from build123d import *

# Parameters (mm, degrees)
F1_DEPTH = 40
F3_DEPTH = 360
F4_R     = 5


with BuildPart() as f1:
    # F0 (on Top) → F1 (new body)
    with BuildSketch(Plane.XY):
        with BuildLine():
            Line((174.920015, 267.026268), (-145.079985, 267.026268))
            ThreePointArc((-145.079985, 267.026268), (-173.364256, 255.310539), (-185.079985, 227.026268))
            Line((-185.079985, 227.026268), (-185.079985, -92.973732))
            ThreePointArc((-185.079985, -92.973732), (-173.364256, -121.258003), (-145.079985, -132.973732))
            Line((-145.079985, -132.973732), (174.920015, -132.973732))
            ThreePointArc((174.920015, -132.973732), (203.204286, -121.258003), (214.920015, -92.973732))
            Line((214.920015, -92.973732), (214.920015, 227.026268))
            ThreePointArc((214.920015, 227.026268), (203.204286, 255.310539), (174.920015, 267.026268))
        make_face()
    extrude(amount=F1_DEPTH)

    # F2 (on face) → F3 (join)
    with BuildSketch(Plane(origin=(0, 0, 0), x_dir=(1, 0, 0), z_dir=(0, 0, -1))):
        with BuildLine():
            ThreePointArc((-145.079985, 62.973732), (-142.151053, 55.902664), (-135.079985, 52.973732))
            Line((-135.079985, 52.973732), (-115.079985, 52.973732))
            ThreePointArc((-115.079985, 52.973732), (-108.008917, 55.902664), (-105.079985, 62.973732))
            Line((-105.079985, 62.973732), (-105.079985, 82.973732))
            ThreePointArc((-105.079985, 82.973732), (-108.008917, 90.0448), (-115.079985, 92.973732))
            Line((-115.079985, 92.973732), (-135.079985, 92.973732))
            ThreePointArc((-135.079985, 92.973732), (-142.151053, 90.0448), (-145.079985, 82.973732))
            Line((-145.079985, 82.973732), (-145.079985, 62.973732))
        make_face()
        with BuildLine():
            Line((-115.079985, -188.623472), (-135.079985, -188.623472))
            ThreePointArc((-135.079985, -188.623472), (-142.151053, -191.552404), (-145.079985, -198.623472))
            Line((-145.079985, -198.623472), (-145.079985, -217.026268))
            ThreePointArc((-145.079985, -217.026268), (-142.151053, -224.097336), (-135.079985, -227.026268))
            Line((-135.079985, -227.026268), (-115.079985, -227.026268))
            ThreePointArc((-115.079985, -227.026268), (-108.008917, -224.097336), (-105.079985, -217.026268))
            Line((-105.079985, -217.026268), (-105.079985, -198.623472))
            ThreePointArc((-105.079985, -198.623472), (-108.008917, -191.552404), (-115.079985, -188.623472))
        make_face()
        with BuildLine():
            ThreePointArc((174.920015, -195.220733), (171.991083, -188.149665), (164.920015, -185.220733))
            Line((164.920015, -185.220733), (144.920015, -185.220733))
            ThreePointArc((144.920015, -185.220733), (137.848947, -188.149665), (134.920015, -195.220733))
            Line((134.920015, -195.220733), (134.920015, -217.026268))
            ThreePointArc((134.920015, -217.026268), (137.848947, -224.097336), (144.920015, -227.026268))
            Line((144.920015, -227.026268), (164.920015, -227.026268))
            ThreePointArc((164.920015, -227.026268), (171.991083, -224.097336), (174.920015, -217.026268))
            Line((174.920015, -217.026268), (174.920015, -195.220733))
        make_face()
        with BuildLine():
            Line((164.920015, 92.973732), (144.920015, 92.973732))
            ThreePointArc((144.920015, 92.973732), (137.848947, 90.0448), (134.920015, 82.973732))
            Line((134.920015, 82.973732), (134.920015, 63.043179))
            ThreePointArc((134.920015, 63.043179), (137.848947, 55.972111), (144.920015, 53.043179))
            Line((144.920015, 53.043179), (164.920015, 53.043179))
            ThreePointArc((164.920015, 53.043179), (171.991083, 55.972111), (174.920015, 63.043179))
            Line((174.920015, 63.043179), (174.920015, 82.973732))
            ThreePointArc((174.920015, 82.973732), (171.991083, 90.0448), (164.920015, 92.973732))
        make_face()
    extrude(amount=F3_DEPTH)

    # F4
    f4_edges = [f1.edges().sort_by_distance(p)[0] for p in [
        (214.920015, 67.026268, 40),
        (203.204286, 255.310539, 40),
        (14.920015, 267.026268, 40),
        (-173.364256, 255.310539, 40),
        (-185.079985, 67.026268, 40),
        (-173.364256, -121.258003, 40),
        (14.920015, -132.973732, 40),
        (203.204286, -121.258003, 40),
    ]]
    fillet(f4_edges, radius=F4_R)


solid = f1.part
For this review, take the finished solid that the model builds, in its own axes (mm). A direction names the side the tool comes from. Coordinates: 2 decimals unless noted, no trailing zeros. Order: outer loops, then holes, each group sorted by start corner. A loop starts at its lowest first (then second) coordinate and runs counter-clockwise, first axis right, second up. Notation, with made-up numbers: (-32, 26) - (-9, 26) arc R22 cw to (-9, 65) - close; hole circle Ø4 at (53, -23.5). An arc over 180 degrees is marked (long way). Answer as CSV lines item,"result". Start each with the question number.
1) To check wall thickness, follow line 1 along X through (y, z) = (213, -328); line 2 along Y through (x, z) = (-123, -45); line 3 along Z through (x, y) = (-116.5, 167). State the ranges of each line that lie inside material, in increasing order. Write a range as [from, to].
2) Draft analysis for pull direction X (two halves, no side actions). For faces 4 (the flat face through (-105.08, 208, -177)), 5 (the flat face through (-185.08, 69, 17)), 6 (the flat face through (13, -132.974, 17)), state which applies: +X half, -X half, draft (parallel to the pull), parting line (faces both ways), or undercut.
3) Add section B-B (x = 77.5). State the section outline as (y, z) points, then the cut area to 3 significant figures.
4) Add section C-C (y = 11). State the section outline as (x, z) points, then the cut area to 3 significant figures.
5) Insertion check: P1, Ø6, axis at x = 156, z = -170, coming from the -Y side; P2, Ø16, axis at y = -73, z = -181, coming from the +X side; P3, Ø24, axis at y = 201, z = -162.5, coming from the -X side. Each pin has a flat end and moves straight along its axis. Give the tip position at first contact, or say it passes through.
6) Machinability: for faces 1 (the flat face through (174.92, -73, -177)), 2 (the flat face through (-145.08, 208, -177)), 3 (the flat face through (-125, -92.974, -177)), which of the approach directions +Z, -Z, +X, -X, +Y, -Y give a long, thin tool a straight path to every point of the face, cutting with its end or side? Answer none if there is none.
7) Add section A-A (z = -122). Count the separate pieces of the cut face and the enclosed holes in it, then the cut area to 3 significant figures.
Result:
1,line 1,"[-145.08, -105.08], [134.92, 174.92]"
1,line 2,"[-92.97, -52.97], [188.62, 227.03]"
1,line 3,"[0, 40]"
2,face 4,"undercut"
2,face 5,"-X half"
2,face 6,"draft"
3,outline,"(-132.97, 0) - (267.03, 0) - (267.03, 35) arc R5 ccw to (262.03, 40) - (-127.97, 40) arc R5 ccw to (-132.97, 35) - close"
3,area,"16,000 mm^2"
4,outline,"(-185.08, 0) - (214.92, 0) - (214.92, 35) arc R5 ccw to (209.92, 40) - (-180.08, 40) arc R5 ccw to (-185.08, 35) - close"
4,area,"16,000 mm^2"
5,P1,"y = -92.97"
5,P2,"x = 174.92"
5,P3,"x = -145.08"
6,face 1,"-Z, +X, +Y, -Y"
6,face 2,"-Z, -X, +Y, -Y"
6,face 3,"-Z, +X, -X, -Y"
7,separate pieces,"4"
7,enclosed holes,"0"
7,area,"6,060 mm^2"
